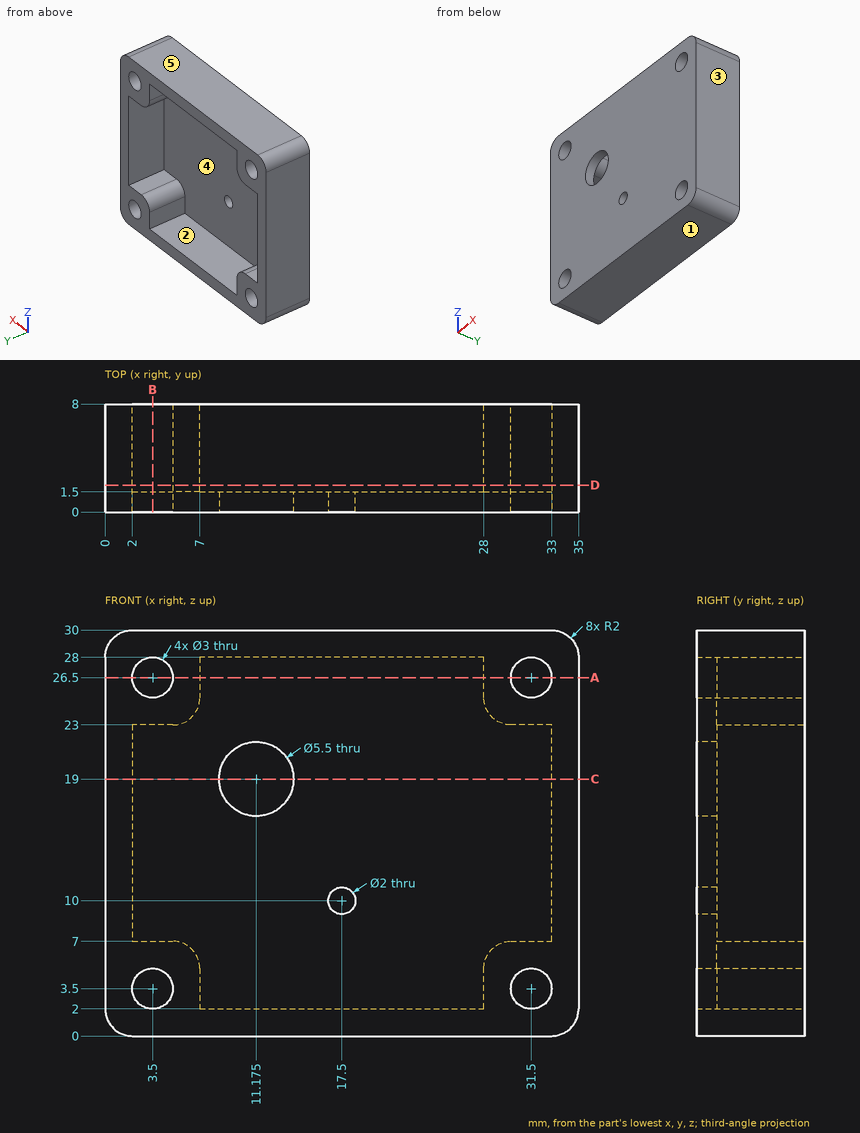
Part print with two shaded views. Sizes in mm from the minimum x, y, z corner. A direction names the side the tool comes from. Give positions to 0.01 mm unless a question says otherwise; leave off trailing zeros. Loops run counter-clockwise (first coordinate to the right, second up) from the corner with the lowest first, then second, coordinate; pieces in that order, holes last. Notation, with made-up numbers: (4, 28) -> (52, 28) arc R11 ccw to (52, 46) -> close; hole circle Ø9 at (20, 50.25). An arc over 180 degrees is marked (long way). One line per question, with ' | ' between items.
Q1. Tool access for the marked faces 4 and 5: list every direction of +Z, -Z, +X, -X, +Y, -Y with a clear straight run to the whole face (end or side of a thin tool).
Filled sheet:
face 4: +Y | face 5: +Z, +X, -X, +Y, -Y
Q2. Cut at A-A, the plane z = 26.5. Write the cut outline in (x, y).
Filled sheet:
outline: (0, 0) -> (2, 0) -> (2, 8) -> (0, 8) -> close; (5, 0) -> (30, 0) -> (30, 8) -> (28, 8) -> (28, 1.5) -> (7, 1.5) -> (7, 8) -> (5, 8) -> close; (33, 0) -> (35, 0) -> (35, 8) -> (33, 8) -> close
Q3. Drop a flat-ended pin along its axis: pin 1 (2.5 mm diameter, centred on x = 17.5, z = 10, fed in from +Y). Give the stop position or say it passes through.
Filled sheet:
pin 1: stops at y = 1.5
Q4. Drill centre lines: line 1 along Z through (x, y) = (31.5, 5); line 2 along X through (y, z) = (3, 27.75); line 3 along Z through (x, y) = (22, 6.75). Where is each one in solid material? Low to high. Write a range as [from, to].
Filled sheet:
line 1: z = [0, 2], [5, 7], [23, 25], [28, 30] | line 2: x = [0, 2.67], [4.33, 7], [28, 30.67], [32.33, 35] | line 3: z = [0, 2], [28, 30]
Q5. Cut at D-D, the plane y = 2. Write the cut outline in (x, z).
Filled sheet:
outline: (0, 2) arc R2 ccw to (2, 0) -> (33, 0) arc R2 ccw to (35, 2) -> (35, 28) arc R2 ccw to (33, 30) -> (2, 30) arc R2 ccw to (0, 28) -> close; hole circle Ø3 at (3.5, 3.5); hole (2, 7) -> (5, 7) arc R2 cw to (7, 5) -> (7, 2) -> (28, 2) -> (28, 5) arc R2 cw to (30, 7) -> (33, 7) -> (33, 23) -> (30, 23) arc R2 cw to (28, 25) -> (28, 28) -> (7, 28) -> (7, 25) arc R2 cw to (5, 23) -> (2, 23) -> close; hole circle Ø3 at (3.5, 26.5); hole circle Ø3 at (31.5, 3.5); hole circle Ø3 at (31.5, 26.5)
Q6. Pull direction X, two halves, no side cores. Call the marked faces 1, 2 and 3: pulls with the +X half, pulls with the -X half, needs draft (parallel to the pull), parting line crosses it, or undercut.
Filled sheet:
face 1: needs draft | face 2: undercut | face 3: pulls with the +X half
Q7. Cut at B-B, the plane x = 3.5. Write the cut outline in (y, z).
Filled sheet:
outline: (0, 0) -> (8, 0) -> (8, 2) -> (0, 2) -> close; (0, 5) -> (8, 5) -> (8, 7) -> (1.5, 7) -> (1.5, 23) -> (8, 23) -> (8, 25) -> (0, 25) -> close; (0, 28) -> (8, 28) -> (8, 30) -> (0, 30) -> close
Q8. Cut at C-C, the plane z = 19. Write the cut outline in (x, y) (1 decimal).
Filled sheet:
outline: (0, 0) -> (8.4, 0) -> (8.4, 1.5) -> (2, 1.5) -> (2, 8) -> (0, 8) -> close; (13.9, 0) -> (35, 0) -> (35, 8) -> (33, 8) -> (33, 1.5) -> (13.9, 1.5) -> close
